For this review, take the finished solid that the model builds, in its own axes (mm). Face numbers are marked on the shaded views. Coordinates: 2 decimals unless noted, no trailing zeros. Write each question's results on one line, items separated by ' | '.
from build123d import *

# Parameters (mm, degrees)
BOSS_EXTRUDE1_DEPTH = 3
SKETCH2_W           = 111.9
SKETCH2_H           = 53.7
BOSS_EXTRUDE2_DEPTH = 1.2
BOSS_EXTRUDE3_DEPTH = 111.9
SKETCH4_W           = 22
SKETCH4_H           = 1.035820464
CUT_EXTRUDE1_DEPTH  = 20
FILLET1_R           = 4
SKETCH5_W           = 25
SKETCH5_H           = 1.236157198
CUT_EXTRUDE2_DEPTH  = 3


with BuildPart() as part:
    # Sketch1 → Boss-Extrude1 (new body)
    with BuildSketch(Plane.XY):
        Polygon((-55.95, 25.65), (-54.75, 25.65), (54.75, 25.65), (54.75, -25.65), (-54.75, -25.65), (-55.95, -25.65), (-55.95, -26.85), (55.95, -26.85), (55.95, 26.85), (-55.95, 26.85), align=None)
    extrude(amount=BOSS_EXTRUDE1_DEPTH)

    # Sketch2 → Boss-Extrude2 (add)
    with BuildSketch(Plane.XY.offset(3)):
        Rectangle(SKETCH2_W, SKETCH2_H)
    extrude(amount=BOSS_EXTRUDE2_DEPTH)

    # Sketch3 → Boss-Extrude3 (add)
    with BuildSketch(Plane(origin=(55.95, 0, 0), x_dir=(0, 0, -1), z_dir=(1, 0, 0))):
        with BuildLine():
            Line((-4.2, -26.886157198), (-5.225151607, -29.702738088))
            Line((-5.225151607, -29.702738088), (-9.225151607, -29.702738088))
            add(Edge.make_bspline(
                [(-4.671449622, 0), (-4.439281188, -15.258416184), (-9.225151607, -29.702738088)],
                knots=[0, 0, 0, 1, 1, 1], degree=2))
            add(Edge.make_bspline(
                [(-4.671449622, 0), (-4.439281188, 15.258416184), (-9.225151607, 29.702738088)],
                knots=[0, 0, 0, 1, 1, 1], degree=2))
            Line((-9.225151607, 29.702738088), (-5.225151607, 29.702738088))
            Line((-5.225151607, 29.702738088), (-4.2, 26.886157198))
            Line((-4.2, 26.886157198), (-4.2, -26.886157198))
        make_face()
    extrude(amount=-BOSS_EXTRUDE3_DEPTH)

    # Sketch4 → Cut-Extrude1 (cut)
    with BuildSketch(Plane(origin=(0, 1.795228959, -4.932351029), x_dir=(-1, 0, 0), z_dir=(0, 0.3420201433256726, -0.939692620785907))):
        with Locations((-16.815363001, 28.380640668)):
            Rectangle(SKETCH4_W, SKETCH4_H)
        with Locations((16.884636999, 28.380640668)):
            Rectangle(SKETCH4_W, SKETCH4_H)
    cut_extrude1 = extrude(amount=-CUT_EXTRUDE1_DEPTH, mode=Mode.SUBTRACT)

    # Mirror1: Cut-Extrude1 across plane
    add(cut_extrude1.mirror(Plane.ZX), mode=Mode.SUBTRACT)

    # Fillet1
    # the kernel refuses this fillet: 4 mm, written as the material it takes off along each edge
    with BuildSketch(Plane(origin=(62.952075382, 29.702738088, 5.225151607), x_dir=(0, 0, 1), z_dir=(-1, 0, 0)), Plane(origin=(62.952075382, -29.702738088, 5.225151607), x_dir=(0, 0.9396926207859048, -0.34202014332567854), z_dir=(-1, 0, 0))) as fillet1_piece_1:
        with BuildLine():
            CenterArc((FILLET1_R * 0.70020753821, -FILLET1_R), FILLET1_R, 90, 70)
            Line((-FILLET1_R * 0.239485082576, -FILLET1_R * 0.657979856674), (0, 0))
            Line((0, 0), (FILLET1_R * 0.70020753821, 0))
        make_face()
    extrude(amount=125.904150764, mode=Mode.SUBTRACT)

    # Sketch5 → Cut-Extrude2 (cut)
    with BuildSketch(Plane(origin=(0, 0, 0), x_dir=(-1, 0, 0), z_dir=(0, 0, -1))):
        with Locations((43.45, -26.268078599)):
            Rectangle(SKETCH5_W, SKETCH5_H)
    extrude(amount=-CUT_EXTRUDE2_DEPTH, mode=Mode.SUBTRACT)


solid = part.part
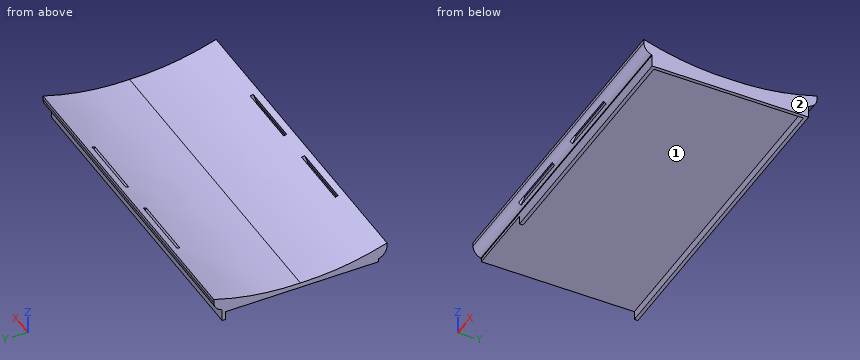
Q1. For pin 1 (0.9 mm diameter, centred on y = 8.5, z = 1, fed in from -X); pin 2 (3.5 mm diameter, centred on x = -20.5, z = 2, fed in from -Y); pin 3 (5 mm diameter, centred on y = 13, z = 8, fed in from +X); pin 4 (1.5 mm diameter, centred on x = 20.5, z = 1.5, fed in from +Y), all flat-tipped, find the tip position at first contact; note any pin that passes through.
Results found:
pin 1: x = 54.75 | pin 2: y = -26.85 | pin 3: through | pin 4: y = 26.85
Q2. Wall thickness on line 1 along Y through (x, z) = (-5.5, 0.5); line 2 along X through (y, z) = (-14, 2.25); line 3 along Y through (x, z) = (15.5, 3.25): over which ranges is each line inside the solid? List them lowest first. Write a range as from..to.
Results found:
line 1: -26.85..-25.65, 25.65..26.85 | line 2: 54.75..55.95 | line 3: -26.85..26.85
Q3. Mouldability with a two-part tool opening along Y and no side actions: class the marked faces 1 and 2 as pulls with the +Y half, pulls with the -Y half, needs draft (parallel to the pull), parting line crosses it, or undercut.
Results found:
face 1: undercut | face 2: needs draft
Q4. Take a section at A-A on x = 25.5. State how many separate pieces and enclosed holes the cut face has, plus the area to 3 significant figures.
Results found:
separate pieces: 3 | enclosed holes: 0 | area: 171 mm2
